Check sheet for the modelled part. Datum: model origin and axes. Units: mm. A direction names the side the tool comes from. Round coordinates to 2 decimals unless told otherwise and drop trailing zeros. Write each loop counter-clockwise with the first axis right and the second up, starting at its lowest first coordinate (ties: lowest second). Pieces come first, ordered by that corner, then holes. Notation, with made-up numbers: (45, -30.75) - (73, -30.75) arc R20 ccw to (73, -3.75) - close; hole circle Ø8 at (78.5, 65.5). An arc over 180 degrees is marked (long way). Use one line per item in the form item = value. Start each with the question number.
1) Draft check along Z on faces 3 (the face through (-4.336, 8.874, 19.524)), 4 (the face through (0, 9, -6)), 5 (the face through (-3, 18, 3)). Enter one of: +Z half, -Z half, draft (parallel to the pull), parting line (faces both ways), or undercut.
2) Section check A-A (z = 0). Record the boundary of the cut face in (x, y).
3) Gauge pin test, flat ends, axial feed: P1, Ø6, axis at y = 4.5, z = -16, coming from the -X side; P2, Ø5, axis at y = 5, z = 4.5, coming from the -X side; P3, Ø1.8, axis at x = 0, y = 4.5, coming from the -Z side. Record the tip position at first contact, or that the pin passes through.
4) Section check D-D (z = 12.5). Record the boundary of the cut face in (x, y), then the cut area to 3 significant figures.
5) Set-up check for faces 1 (the face through (-3, 0, 3)), 2 (the face through (-8.675, 8.874, -3.422)): record each of +Z, -Z, +X, -X, +Y, -Y from which the full face is reachable in a straight line by a thin tool's end or side.
6) Scan lines: probe 1 along X at (y, z) = (8.5, -5); probe 2 along Z at (x, y) = (6.5, 6). Record each from-to range of solid material in increasing order.
7) Section check B-B (x = 0). Record the boundary of the cut face in (y, z), then the cut area to 3 significant figures.
8) Section check C-C (x = -5). Record the boundary of the cut face in (y, z), then the cut area to 3 significant figures.
from build123d import *

# Parameters (mm, degrees)
SKETCH_2_R      = 20
SKETCH_2_R_2    = 2
EXTRUDE_1_DEPTH = 18


with BuildPart() as part:
    # 草图2 → 凸台-拉伸1 (new body)
    with BuildSketch(Plane(origin=(0, 0, 0), x_dir=(1, 0, 0), z_dir=(0, 1, 0))):
        Circle(SKETCH_2_R)
        with Locations((-5, 5)):
            Circle(SKETCH_2_R_2, mode=Mode.SUBTRACT)
        with Locations((5, 5)):
            Circle(SKETCH_2_R_2, mode=Mode.SUBTRACT)
        with Locations((5, -5)):
            Circle(SKETCH_2_R_2, mode=Mode.SUBTRACT)
        with Locations((-5, -5)):
            Circle(SKETCH_2_R_2, mode=Mode.SUBTRACT)
        with BuildLine():
            Line((-8.445719569, 7.031506006), (-13.415371808, 12.001158246))
            ThreePointArc((-13.415371808, 12.001158246), (-18, 0), (-13.415371808, -12.001158246))
            Line((-13.415371808, -12.001158246), (-8.445719569, -7.031506006))
            ThreePointArc((-8.445719569, -7.031506006), (-8.69551813, -3.469266271), (-6, -1.127016654))
            Line((-6, -1.127016654), (-6, 1.127016654))
            ThreePointArc((-6, 1.127016654), (-8.69551813, 3.469266271), (-8.445719569, 7.031506006))
        make_face(mode=Mode.SUBTRACT)
        with BuildLine():
            Line((-12.001158246, 13.415371808), (-7.031506006, 8.445719569))
            ThreePointArc((-7.031506006, 8.445719569), (-3.469266271, 8.69551813), (-1.127016654, 6))
            Line((-1.127016654, 6), (1.127016654, 6))
            ThreePointArc((1.127016654, 6), (3.469266271, 8.69551813), (7.031506006, 8.445719569))
            Line((7.031506006, 8.445719569), (12.001158246, 13.415371808))
            ThreePointArc((12.001158246, 13.415371808), (0, 18), (-12.001158246, 13.415371808))
        make_face(mode=Mode.SUBTRACT)
        with BuildLine():
            Line((13.415371808, 12.001158246), (8.445719569, 7.031506006))
            ThreePointArc((8.445719569, 7.031506006), (8.69551813, 3.469266271), (6, 1.127016654))
            Line((6, 1.127016654), (6, -1.127016654))
            ThreePointArc((6, -1.127016654), (8.69551813, -3.469266271), (8.445719569, -7.031506006))
            Line((8.445719569, -7.031506006), (13.415371808, -12.001158246))
            ThreePointArc((13.415371808, -12.001158246), (18, 0), (13.415371808, 12.001158246))
        make_face(mode=Mode.SUBTRACT)
        with BuildLine():
            Line((12.001158246, -13.415371808), (7.031506006, -8.445719569))
            ThreePointArc((7.031506006, -8.445719569), (3.469266271, -8.69551813), (1.127016654, -6))
            Line((1.127016654, -6), (-1.127016654, -6))
            ThreePointArc((-1.127016654, -6), (-3.469266271, -8.69551813), (-7.031506006, -8.445719569))
            Line((-7.031506006, -8.445719569), (-12.001158246, -13.415371808))
            ThreePointArc((-12.001158246, -13.415371808), (0, -18), (12.001158246, -13.415371808))
        make_face(mode=Mode.SUBTRACT)
        with BuildLine():
            Line((-1.127016654, 4), (1.127016654, 4))
            ThreePointArc((1.127016654, 4), (2.171572875, 2.171572875), (4, 1.127016654))
            Line((4, 1.127016654), (4, -1.127016654))
            ThreePointArc((4, -1.127016654), (2.171572875, -2.171572875), (1.127016654, -4))
            Line((1.127016654, -4), (-1.127016654, -4))
            ThreePointArc((-1.127016654, -4), (-2.171572875, -2.171572875), (-4, -1.127016654))
            Line((-4, -1.127016654), (-4, 1.127016654))
            ThreePointArc((-4, 1.127016654), (-2.171572875, 2.171572875), (-1.127016654, 4))
        make_face(mode=Mode.SUBTRACT)
    extrude(amount=EXTRUDE_1_DEPTH)


solid = part.part
Results are:
q1.face_3 = parting line
q1.face_4 = undercut
q1.face_5 = draft
q2.outline = (-20, 0) - (-18, 0) - (-18, 18) - (-20, 18) - close; (-6, 0) - (-4, 0) - (-4, 18) - (-6, 18) - close; (4, 0) - (6, 0) - (6, 18) - (4, 18) - close; (18, 0) - (20, 0) - (20, 18) - (18, 18) - close
q3.P1 = -15.2
q3.P2 = -19.9
q3.P3 = -20
q4.outline = (-15.61, 0) - (-11.09, 0) - (-11.09, 18) - (-15.61, 18) - close; (11.09, 0) - (15.61, 0) - (15.61, 18) - (11.09, 18) - close
q4.area = 163 mm²
q5.face_1 = +Z, -Z, +X, -X, -Y
q5.face_2 = +Y, -Y
q6.probe_1 = -19.36 to -17.29, -9 to -7, -3 to 3, 7 to 9, 17.29 to 19.36
q6.probe_2 = -18.91 to -16.79, -8.71 to -6.32, -3.68 to -1.29, 1.29 to 3.68, 6.32 to 8.71, 16.79 to 18.91
q7.outline = (0, -20) - (18, -20) - (18, -18) - (0, -18) - close; (0, -6) - (18, -6) - (18, -4) - (0, -4) - close; (0, 4) - (18, 4) - (18, 6) - (0, 6) - close; (0, 18) - (18, 18) - (18, 20) - (0, 20) - close
q7.area = 144 mm²
q8.outline = (0, -19.36) - (18, -19.36) - (18, -17.29) - (0, -17.29) - close; (0, -9) - (18, -9) - (18, -7) - (0, -7) - close; (0, -3) - (18, -3) - (18, 3) - (0, 3) - close; (0, 7) - (18, 7) - (18, 9) - (0, 9) - close; (0, 17.29) - (18, 17.29) - (18, 19.36) - (0, 19.36) - close
q8.area = 255 mm²
